```python
from build123d import *

# Parameters (mm, degrees)
SKETCH4_R           = 17.5
SKETCH4_R_2         = 2.1
BOSS_EXTRUDE1_DEPTH = 2
BOSS_EXTRUDE2_DEPTH = 4
SKETCH5_R           = 2.1
CUT_EXTRUDE2_DEPTH  = 5


with BuildPart() as part:
    # Sketch4 → Boss-Extrude1 (new body)
    with BuildSketch(Plane(origin=(0, 0, 0), x_dir=(1, 0, 0), z_dir=(0, 1, 0))):
        Circle(SKETCH4_R)
        Circle(SKETCH4_R_2, mode=Mode.SUBTRACT)
    extrude(amount=BOSS_EXTRUDE1_DEPTH)

    # Sketch1 → Boss-Extrude2 (add)
    with BuildSketch(Plane(origin=(0, 0, 0), x_dir=(1, 0, 0), z_dir=(0, 1, 0))):
        with BuildLine():
            Line((-8.26, 15), (8.26, 15))
            ThreePointArc((8.26, 15), (0, 6.74), (-8.26, 15))
        make_face()
        with BuildLine():
            Line((15, 8.26), (15, -8.26))
            ThreePointArc((15, -8.26), (6.74, 0), (15, 8.26))
        make_face()
        with BuildLine():
            Line((8.26, -15), (-8.26, -15))
            ThreePointArc((-8.26, -15), (0, -6.74), (8.26, -15))
        make_face()
        with BuildLine():
            Line((-15, -8.26), (-15, 8.26))
            ThreePointArc((-15, 8.26), (-6.74, 0), (-15, -8.26))
        make_face()
    extrude(amount=BOSS_EXTRUDE2_DEPTH)

    # Sketch5 → Cut-Extrude2 (cut, through all)
    with BuildSketch(Plane(origin=(0, 4, 0), x_dir=(1, 0, 0), z_dir=(0, 1, 0))):
        with Locations((0, 10.87)):
            Circle(SKETCH5_R)
        with Locations((10.87, 0)):
            Circle(SKETCH5_R)
        with Locations((0, -10.87)):
            Circle(SKETCH5_R)
        with Locations((-10.87, 0)):
            Circle(SKETCH5_R)
    extrude(amount=-CUT_EXTRUDE2_DEPTH, mode=Mode.SUBTRACT)


solid = part.part
```
Could you check a few things on this model? Use its own coordinates, in mm. A direction names the side the tool comes from. Give positions to 0.01 mm unless a question says otherwise; leave off trailing zeros. Loops run counter-clockwise (first coordinate to the right, second up) from the corner with the lowest first, then second, coordinate; pieces in that order, holes last. Notation, with made-up numbers: (-36.5, 80) - (-2.5, 80) arc R28 ccw to (-2.5, 114) - close; hole circle Ø11 at (61.5, 66.5). An arc over 180 degrees is marked (long way). Answer in a Markdown table with one row per item. Add a question column.
Q1. We'd pull the mould along Z, two halves only. Please class faces 1 (the face through (-15, 3, 0)), 2 (the face through (6.74, 2.99, 0.18)), 3 (the face through (0, 3, 15)), 4 (the face through (-0.273, 2.028, -12.952)): +Z half, -Z half, draft (parallel to the pull), parting line (faces both ways), or undercut.
Q2. Which directions (+Z, -Z, +X, -X, +Y, -Y) give clear straight access to the entire face, cutting with the end or side of a thin tool? Please do faces 5 (the face through (15, 3, 0)), 6 (the face through (0.18, 2.99, -6.74)), 7 (the face through (0, 3, -15)).
Q3. If we section it at B-B (x = 0): List the corners of the cut face in (y, z) for me.
Q4. If we section it at A-A (y = 2.95): List the corners of the cut face in (x, z) for me, plus the area to 3 significant figures.
Q5. If we section it at D-D (x = -11): List the corners of the cut face in (y, z) for me.
Q6. If we section it at C-C (z = -11.5): List the corners of the cut face in (x, y) for me.
Q7. For pin 1 (5 mm diameter, centred on x = -10.87, z = 0, fed in from -Y); pin 2 (1 mm diameter, centred on x = -2, y = 1.5, fed in from -Z); pin 3 (1 mm diameter, centred on y = 3, z = 1, fed in from -X); pin 4 (1.6 mm diameter, centred on y = 3.5, z = 3.5, fed in from +X), each with a flat end and sliding along its axis, tell me the tip position at first contact or that it passes through.
Q8. Please list where these lines run through material, in increasing order: L1, parallel to X at y = 1.1, z = 0; L2, parallel to X at y = 2.9, z = 0. Write a range as from..to.
The answers:
| question | item | result |
|---|---|---|
| 1 | face 1 | draft |
| 1 | face 2 | undercut |
| 1 | face 3 | +Z half |
| 1 | face 4 | undercut |
| 2 | face 5 | +Z, -Z, +X, +Y |
| 2 | face 6 | +Y |
| 2 | face 7 | -Z, +X, -X, +Y |
| 3 | outline | (0, -17.5) - (2, -17.5) - (2, -15) - (4, -15) - (4, -12.97) - (0, -12.97) - close; (0, -8.77) - (4, -8.77) - (4, -6.74) - (2, -6.74) - (2, -2.1) - (0, -2.1) - close; (0, 2.1) - (2, 2.1) - (2, 6.74) - (4, 6.74) - (4, 8.77) - (0, 8.77) - close; (0, 12.97) - (4, 12.97) - (4, 15) - (2, 15) - (2, 17.5) - (0, 17.5) - close |
| 4 | outline | (-15, -8.26) arc R8.26 ccw to (-15, 8.26) - close; (-8.26, -15) - (8.26, -15) arc R8.26 ccw to start; (-8.26, 15) arc R8.26 ccw to (8.26, 15) - close; (15, -8.26) - (15, 8.26) arc R8.26 ccw to start; hole circle Ø4.2 at (-10.87, 0); hole circle Ø4.2 at (0, -10.87); hole circle Ø4.2 at (0, 10.87); hole circle Ø4.2 at (10.87, 0) |
| 4 | area | 373 mm^2 |
| 5 | outline | (0, -13.61) - (2, -13.61) - (2, -7.23) - (4, -7.23) - (4, -2.1) - (0, -2.1) - close; (0, 2.1) - (4, 2.1) - (4, 7.23) - (2, 7.23) - (2, 13.61) - (0, 13.61) - close |
| 6 | outline | (-13.19, 0) - (-2, 0) - (-2, 4) - (-7.48, 4) - (-7.48, 2) - (-13.19, 2) - close; (2, 0) - (13.19, 0) - (13.19, 2) - (7.48, 2) - (7.48, 4) - (2, 4) - close |
| 7 | pin 1 | stops at y = 0 |
| 7 | pin 2 | stops at z = -17.44 |
| 7 | pin 3 | stops at x = -15 |
| 7 | pin 4 | stops at x = 15 |
| 8 | L1 | x = -17.5..-12.97, -8.77..-2.1, 2.1..8.77, 12.97..17.5 |
| 8 | L2 | x = -15..-12.97, -8.77..-6.74, 6.74..8.77, 12.97..15 |
